Here's how the part is built. I have some questions about the finished solid (model axes, mm). Round coordinates to 2 decimals unless told otherwise and drop trailing zeros. Order: outer loops, then holes, each group sorted by start corner. A loop starts at its lowest first (then second) coordinate and runs counter-clockwise, first axis right, second up.
```python
from build123d import *

# Parameters (mm, degrees)
SKETCH1_W               = 40
SKETCH1_H               = 40
BOSS_EXTRUDE1_DEPTH     = 6
F_6_0MM_DOWEL_HOLE1_D   = 6
SKETCH5_R               = 12.5
CUT_EXTRUDE1_DEPTH      = 57.885850613
TAP_DRILL_FOR_M4_TAP1_D = 3.3


with BuildPart() as part:
    # Sketch1 → Boss-Extrude1 (new body)
    with BuildSketch(Plane.XY):
        with Locations((20, 20)):
            Rectangle(SKETCH1_W, SKETCH1_H)
    extrude(amount=BOSS_EXTRUDE1_DEPTH)

    # Ø6.0mm Dowel Hole1 (through all)
    with Locations(Plane.XY.offset(6)):
        with Locations((5.857864376, 5.857864376), (5.857864376, 34.142135624), (34.142135624, 34.142135624), (34.142135624, 5.857864376)):
            Hole(F_6_0MM_DOWEL_HOLE1_D / 2)

    # Sketch5 → Cut-Extrude1 (cut, through all)
    with BuildSketch(Plane.XY.offset(6)):
        with Locations((20, 20)):
            Circle(SKETCH5_R)
    extrude(amount=-CUT_EXTRUDE1_DEPTH, mode=Mode.SUBTRACT)

    # Tap Drill for M4 Tap1 (through all)
    with Locations(Plane.XY.offset(6)):
        with Locations((4.5, 20), (20, 35.5), (35.5, 20), (20, 4.5)):
            Hole(TAP_DRILL_FOR_M4_TAP1_D / 2)


solid = part.part
```
1) We'd pull the mould along X, two halves only. Please class faces 1 (the flat face through (0, 20, 3)), 2 (the flat face through (11, 29, 0)), 3 (the cylindrical face through (32.53, 36.67, 2.96)): +X half, -X half, draft (parallel to the pull), parting line (faces both ways), or undercut.
2) I'm going to push flat-ended pins straight in: pin 1 (1 mm diameter, centred on x = 14, z = 2.5, fed in from -Y); pin 2 (8 mm diameter, centred on x = 16, y = 16, fed in from +Z). Where does each tip first touch, or does it pass through?
3) If we section it at A-A (y = 20): Write out the boundary of the cut face in (x, z).
4) If we section it at D-D (x = 23): Write out the boundary of the cut face in (y, z), plus the area to 3 significant figures.
5) If we section it at B-B (y = 24.5): Write out the boundary of the cut face in (x, z), plus the area to 3 significant figures.
6) If we section it at C-C (x = 35.5): Write out the boundary of the cut face in (y, z).
7) I need wall thicknesses on line 1 (Y direction, x = 20, z = 4.4); line 2 (X direction, y = 5, z = 1.75); line 3 (Y direction, x = 6.5, z = 1.65). Which ranges of each line are inside material? Lowest first, please.
Solutions:
1. face 1: -X half
1. face 2: draft
1. face 3: undercut
2. pin 1: stops at y = 0
2. pin 2: passes through
3. outline: (0, 0) - (2.85, 0) - (2.85, 6) - (0, 6) - close; (6.15, 0) - (7.5, 0) - (7.5, 6) - (6.15, 6) - close; (32.5, 0) - (33.85, 0) - (33.85, 6) - (32.5, 6) - close; (37.15, 0) - (40, 0) - (40, 6) - (37.15, 6) - close
4. outline: (0, 0) - (7.87, 0) - (7.87, 6) - (0, 6) - close; (32.13, 0) - (40, 0) - (40, 6) - (32.13, 6) - close
4. area: 94.4 mm2
5. outline: (0, 0) - (8.34, 0) - (8.34, 6) - (0, 6) - close; (31.66, 0) - (40, 0) - (40, 6) - (31.66, 6) - close
5. area: 100 mm2
6. outline: (0, 0) - (3.18, 0) - (3.18, 6) - (0, 6) - close; (8.53, 0) - (18.35, 0) - (18.35, 6) - (8.53, 6) - close; (21.65, 0) - (31.47, 0) - (31.47, 6) - (21.65, 6) - close; (36.82, 0) - (40, 0) - (40, 6) - (36.82, 6) - close
7. line 1: y = 0 to 2.85, 6.15 to 7.5, 32.5 to 33.85, 37.15 to 40
7. line 2: x = 0 to 2.98, 8.73 to 18.43, 21.57 to 31.27, 37.02 to 40
7. line 3: y = 0 to 2.93, 8.79 to 31.21, 37.07 to 40
